from build123d import *

# Parameters (mm, degrees)
ESQUISSE3_W                                 = 44
ESQUISSE3_H                                 = 44
BOSS_EXTRU_1_DEPTH                          = 2
SKETCH_HOLES_R                              = 0.5
CUT_EXTRUDE_HOLES_DEPTH                     = 3
FRAISAGE_POUR_VIS_T_TE_FRAIS_E_M21_AT_COUNT = 2
FRAISAGE_POUR_VIS_T_TE_FRAIS_E_M21_AT_PITCH = 39
FRAISAGE_POUR_VIS_T_TE_FRAIS_E_M21_2_COUNT  = 2
FRAISAGE_POUR_VIS_T_TE_FRAIS_E_M21_2_PITCH  = 55.154328933
FRAISAGE_POUR_VIS_T_TE_FRAIS_E_M21_3_COUNT  = 2
FRAISAGE_POUR_VIS_T_TE_FRAIS_E_M21_3_PITCH  = 39


with BuildPart() as part:
    # Esquisse3 → Boss.-Extru.1 (new body)
    with BuildSketch(Plane(origin=(0, 0, 0), x_dir=(0, 1, 0), z_dir=(0, 0, 1))):
        Rectangle(ESQUISSE3_W, ESQUISSE3_H)
    extrude(amount=BOSS_EXTRU_1_DEPTH)

    # Sketch_Holes → Cut_Extrude_Holes (cut, through all)
    with BuildSketch(Plane.XY.offset(2)):
        with Locations((-10.067654011, 4.160184375)):
            Circle(SKETCH_HOLES_R)
    extrude(amount=-CUT_EXTRUDE_HOLES_DEPTH, mode=Mode.SUBTRACT)

    # Esquisse5 → Fraisage pour vis à tête fraisée M21 (revolve, cut)
    with BuildSketch(Plane(origin=(19.5, -19.5, 2), x_dir=(0, -1, 0), z_dir=(1, 0, 0))):
        Polygon((0, 0), (0, 2), (1.2, 2), (1.2, 1), (2.2, 0), align=None)
    fraisage_pour_vis_t_te_frais_e_m21 = revolve(axis=Axis((19.5, -19.5, 8.35), (0, 0, -1)), mode=Mode.SUBTRACT)

    # Fraisage pour vis à tête fraisée M21 at: Fraisage pour vis à tête fraisée M21 ×2
    with Locations(*[(-i * FRAISAGE_POUR_VIS_T_TE_FRAIS_E_M21_AT_PITCH, 0, 0) for i in range(1, FRAISAGE_POUR_VIS_T_TE_FRAIS_E_M21_AT_COUNT)]):
        add(fraisage_pour_vis_t_te_frais_e_m21, mode=Mode.SUBTRACT)

    # Fraisage pour vis _ t_te frais_e M21 2: Fraisage pour vis à tête fraisée M21 ×2
    with Locations(*[Vector(-0.707106781, 0.707106781, 0) * (i * FRAISAGE_POUR_VIS_T_TE_FRAIS_E_M21_2_PITCH) for i in range(1, FRAISAGE_POUR_VIS_T_TE_FRAIS_E_M21_2_COUNT)]):
        add(fraisage_pour_vis_t_te_frais_e_m21, mode=Mode.SUBTRACT)

    # Fraisage pour vis _ t_te frais_e M21 3: Fraisage pour vis à tête fraisée M21 ×2
    with Locations(*[(0, i * FRAISAGE_POUR_VIS_T_TE_FRAIS_E_M21_3_PITCH, 0) for i in range(1, FRAISAGE_POUR_VIS_T_TE_FRAIS_E_M21_3_COUNT)]):
        add(fraisage_pour_vis_t_te_frais_e_m21, mode=Mode.SUBTRACT)


solid = part.part
Can you work these out from the model? Positions are in its coordinate system, mm. Give positions to 0.01 mm unless a question says otherwise; leave off trailing zeros. Loops run counter-clockwise (first coordinate to the right, second up) from the corner with the lowest first, then second, coordinate; pieces in that order, holes last. Notation, with made-up numbers: (75, -36) - (89, -36) arc R8 cw to (89, -21) - close; hole circle Ø7 at (29, 59). An arc over 180 degrees is marked (long way). Answer as a JSON object with one key per item and string values.
Q1. If I drill on L1, parallel to Y at x = 19.5, z = 0.55; L2, parallel to X at y = -20, z = 1.15, over which ranges is the centre line in solid material (lowest first)?
Geometry says:
{"L1": "-22 to -20.7, -18.3 to 18.3, 20.7 to 22", "L2": "-22 to -20.75, -18.25 to 18.25, 20.75 to 22"}
Q2. Imagine slicing it at C-C on z = 1.45. Write out the boundary of the cut face in (x, y), plus the area to 3 significant figures.
Geometry says:
{"outline": "(-22, -22) - (22, -22) - (22, 22) - (-22, 22) - close; hole circle Ø3.3 at (-19.5, -19.5); hole circle Ø3.3 at (-19.5, 19.5); hole circle Ø1 at (-10.07, 4.16); hole circle Ø3.3 at (19.5, -19.5); hole circle Ø3.3 at (19.5, 19.5)", "area": "1,900 mm²"}
Q3. Will these pins go through, and if not, where does the flat tip stop? P1, Ø3, axis at x = -19.5, y = 19.5, coming from the +Z side; P2, Ø4, axis at x = -19.5, y = -19.5, coming from the +Z side.
Geometry says:
{"P1": "z = 1.3", "P2": "z = 1.8"}
Q4. If we mould it in two halves opening along X, with no side actions, what happens to faces 1 (the flat face through (0, 0, 2)), 2 (the cylindrical face through (-18.435, 18.946, 0.507)), 3 (the flat face through (-22, 0, 1))? For each: pulls with the +X half, pulls with the -X half, needs draft (parallel to the pull), parting line crosses it, or undercut.
Geometry says:
{"face 1": "needs draft", "face 2": "undercut", "face 3": "pulls with the -X half"}
Q5. Imagine slicing it at A-A on y = 19.5. Write out the boundary of the cut face in (x, z).
Geometry says:
{"outline": "(-22, 0) - (-20.7, 0) - (-20.7, 1) - (-21.7, 2) - (-22, 2) - close; (-18.3, 0) - (18.3, 0) - (18.3, 1) - (17.3, 2) - (-17.3, 2) - (-18.3, 1) - close; (20.7, 0) - (22, 0) - (22, 2) - (21.7, 2) - (20.7, 1) - close"}
